```python
from build123d import *

# Parameters (mm, degrees)
SKETCH1_R               = 63.5
BOSS_EXTRUDE1_DEPTH     = 12.7
SKETCH2_R               = 44.45
BOSS_EXTRUDE2_DEPTH     = 6.35
SKETCH3_R               = 24.13
CUT_EXTRUDE1_DEPTH      = 1
CUT_EXTRUDE1_DEPTH_BACK = 20.05
SKETCH4_R               = 2.0955
CUT_EXTRUDE2_DEPTH      = 20.05


with BuildPart() as part:
    # Sketch1 → Boss-Extrude1 (new body)
    with BuildSketch(Plane(origin=(0, 0, 0), x_dir=(1, 0, 0), z_dir=(0, 1, 0))):
        Circle(SKETCH1_R)
    extrude(amount=BOSS_EXTRUDE1_DEPTH)

    # Sketch2 → Boss-Extrude2 (add)
    with BuildSketch(Plane(origin=(0, 12.7, 0), x_dir=(1, 0, 0), z_dir=(0, 1, 0))):
        Circle(SKETCH2_R)
    extrude(amount=BOSS_EXTRUDE2_DEPTH)

    # Sketch3 → Cut-Extrude1 (cut, two sides)
    with BuildSketch(Plane(origin=(0, 19.05, 0), x_dir=(1, 0, 0), z_dir=(0, 1, 0))) as cut_extrude1_sk:
        Circle(SKETCH3_R)
    extrude(amount=CUT_EXTRUDE1_DEPTH, mode=Mode.SUBTRACT)
    extrude(cut_extrude1_sk.sketch, amount=-CUT_EXTRUDE1_DEPTH_BACK, mode=Mode.SUBTRACT)

    # Sketch4 → Cut-Extrude2 (cut, through all)
    with BuildSketch(Plane.XZ):
        with Locations((0, -58.42)):
            Circle(SKETCH4_R)
        with Locations((-29.21, -50.593204089)):
            Circle(SKETCH4_R)
        with Locations((-50.593204089, -29.21)):
            Circle(SKETCH4_R)
        with Locations((-58.42, 0)):
            Circle(SKETCH4_R)
        with Locations((-50.593204089, 29.21)):
            Circle(SKETCH4_R)
        with Locations((-29.21, 50.593204089)):
            Circle(SKETCH4_R)
        with Locations((0, 58.42)):
            Circle(SKETCH4_R)
        with Locations((29.21, 50.593204089)):
            Circle(SKETCH4_R)
        with Locations((50.593204089, 29.21)):
            Circle(SKETCH4_R)
        with Locations((58.42, 0)):
            Circle(SKETCH4_R)
        with Locations((50.593204089, -29.21)):
            Circle(SKETCH4_R)
        with Locations((29.21, -50.593204089)):
            Circle(SKETCH4_R)
    extrude(amount=-CUT_EXTRUDE2_DEPTH, mode=Mode.SUBTRACT)


solid = part.part
```
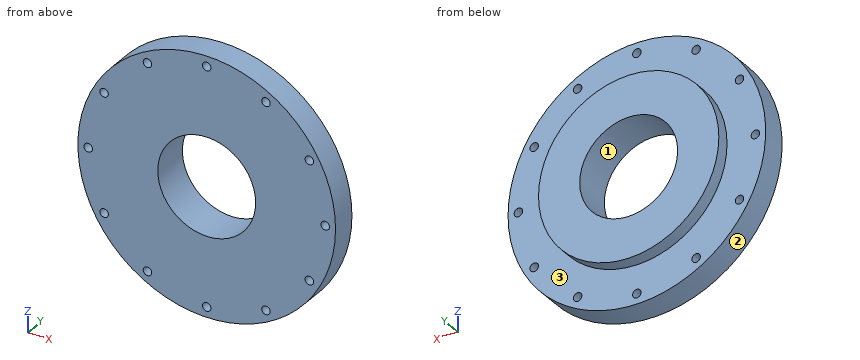
The model under review builds one solid part; all positions refer to its coordinate system, in mm. Face numbers are marked on the shaded views. Give positions to 0.01 mm unless a question says otherwise; leave off trailing zeros. Write each loop counter-clockwise with the first axis right and the second up, starting at its lowest first coordinate (ties: lowest second). Pieces come first, ordered by that corner, then holes. Notation, with made-up numbers: M 72.5,19.5 L 101.5,19.5 A20 cw 101.5,29.5 Z; hole C 41.5,-22.75 d6. An arc over 180 degrees is marked long. Answer in a Markdown table with one row per item.
Item 1: For P1, Ø6.5, axis at x = 58.42, z = 0, coming from the +Y side; P2, Ø5, axis at x = 44.5, y = 8.5, coming from the +Z side; P3, Ø5, axis at x = -15.5, y = 13, coming from the +Z side, all flat-tipped, find the tip position at first contact; note any pin that passes through.
Check sheet entries:
| item | result |
|---|---|
| P1 | y = 12.7 |
| P2 | z = 47.63 |
| P3 | z = 62.15 |
Item 2: Add section B-B on x = 0. Give the boundary of the cut face in (y, z), plus the area to 3 significant figures.
Check sheet entries:
| item | result |
|---|---|
| outline | M 0,-63.5 L 12.7,-63.5 L 12.7,-60.52 L 0,-60.52 Z; M 0,-56.32 L 12.7,-56.32 L 12.7,-44.45 L 19.05,-44.45 L 19.05,-24.13 L 0,-24.13 Z; M 0,24.13 L 19.05,24.13 L 19.05,44.45 L 12.7,44.45 L 12.7,56.32 L 0,56.32 Z; M 0,60.52 L 12.7,60.52 L 12.7,63.5 L 0,63.5 Z |
| area | 1,150 mm2 |
Item 3: Draft analysis for pull direction X (two halves, no side actions). For the marked faces 1, 2 and 3, state which applies: +X half, -X half, draft (parallel to the pull), parting line (faces both ways), or undercut.
Check sheet entries:
| item | result |
|---|---|
| face 1 | undercut |
| face 2 | parting line |
| face 3 | draft |
Item 4: Add section D-D on y = 6.5. State how many separate pieces and enclosed holes the cut face has, plus the area to 3 significant figures.
Check sheet entries:
| item | result |
|---|---|
| separate pieces | 1 |
| enclosed holes | 13 |
| area | 10,700 mm2 |
Item 5: For line 1 along X through (y, z) = (4.25, -49); line 2 along Z through (x, y) = (-29.21, 7.5); line 3 along X through (y, z) = (5.25, 50.5), list the stretches that pass through material, from the lowest coordinate up.
Check sheet entries:
| item | result |
|---|---|
| line 1 | -40.39 to -30.57, -27.85 to 27.85, 30.57 to 40.39 |
| line 2 | -56.38 to -52.69, -48.5 to 48.5, 52.69 to 56.38 |
| line 3 | -38.5 to -31.3, -27.12 to 27.12, 31.3 to 38.5 |
Item 6: Add section A-A on z = 20.5. Give the boundary of the cut face in (x, y).
Check sheet entries:
| item | result |
|---|---|
| outline | M -60.1,0 L -12.73,0 L -12.73,19.05 L -39.44,19.05 L -39.44,12.7 L -60.1,12.7 Z; M 12.73,0 L 60.1,0 L 60.1,12.7 L 39.44,12.7 L 39.44,19.05 L 12.73,19.05 Z |
Item 7: Add section C-C on x = 29.21. Give the boundary of the cut face in (y, z).
Check sheet entries:
| item | result |
|---|---|
| outline | M 0,-56.38 L 12.7,-56.38 L 12.7,-52.69 L 0,-52.69 Z; M 0,-48.5 L 12.7,-48.5 L 12.7,-33.5 L 19.05,-33.5 L 19.05,33.5 L 12.7,33.5 L 12.7,48.5 L 0,48.5 Z; M 0,52.69 L 12.7,52.69 L 12.7,56.38 L 0,56.38 Z |
